Model file for the job. Use its own axes, mm. Face numbers are marked on the shaded views. A direction names the side the tool comes from. Round coordinates to 2 decimals unless told otherwise and drop trailing zeros. Write each loop counter-clockwise with the first axis right and the second up, starting at its lowest first coordinate (ties: lowest second). Pieces come first, ordered by that corner, then holes. Notation, with made-up numbers: (41.25, 45.25) - (75.25, 45.25) arc R26 cw to (75.25, 81.25) - close; hole circle Ø2 at (87, -18). An arc over 180 degrees is marked (long way). One line per item, written item: value.
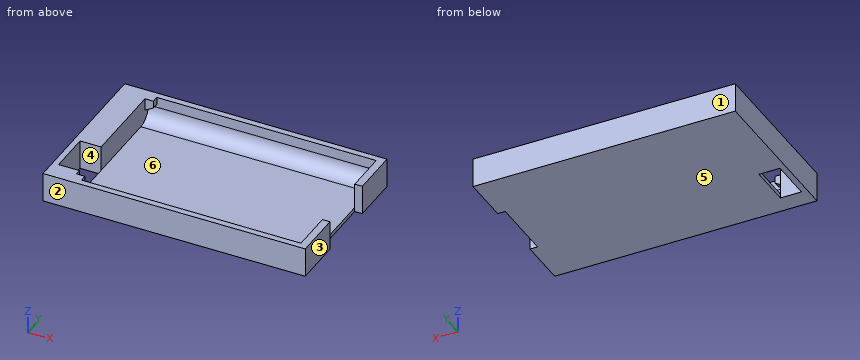
from build123d import *

# Parameters (mm, degrees)
SKETCH2_W                 = 62.4
SKETCH2_H                 = 38
BOSS_EXTRUDE1_DEPTH       = 7
CUT_EXTRUDE1_DEPTH        = 27.1
SKETCH4_W                 = 1.8
SKETCH4_H                 = 15
FORFINGER_DEPTH           = 40.143965052
SKETCH5_W                 = 2
SKETCH5_H                 = 2.9
BOSS_EXTRUDE2_DEPTH       = 1.6
CHAMFER1_SIZE2            = 1.154700538
CHAMFER1_SIZE             = 2
CHAMFER1_OF_MIRROR1_SIZE2 = 1.154700538
CHAMFER1_OF_MIRROR1_SIZE  = 2
SKETCH6_W                 = 5
SKETCH6_H                 = 10
CUT_EXTRUDE3_DEPTH        = 40.143965052


with BuildPart() as part:
    # Sketch2 → Boss-Extrude1 (new body)
    with BuildSketch(Plane.XY):
        with Locations((-2.3, 0)):
            Rectangle(SKETCH2_W, SKETCH2_H)
    extrude(amount=BOSS_EXTRUDE1_DEPTH)

    # Sketch3 → Cut-Extrude1 (cut, symmetric)
    with BuildSketch(Plane(origin=(0, 0, 0), x_dir=(0, 0, -1), z_dir=(1, 0, 0))):
        with BuildLine():
            Line((-8, 17.5), (-4.5, 17.5))
            ThreePointArc((-4.5, 17.5), (-2.025126266, 16.474873734), (-1, 14))
            Line((-1, 14), (-1, -14))
            ThreePointArc((-1, -14), (-2.025126266, -16.474873734), (-4.5, -17.5))
            Line((-4.5, -17.5), (-8, -17.5))
            Line((-8, -17.5), (-8, 17.5))
        make_face()
    extrude(amount=CUT_EXTRUDE1_DEPTH, both=True, mode=Mode.SUBTRACT)

    # Sketch4 → ForFinger (cut, through all)
    with BuildSketch(Plane.XY.offset(7)):
        with Locations((28, 0)):
            Rectangle(SKETCH4_W, SKETCH4_H)
    extrude(amount=-FORFINGER_DEPTH, mode=Mode.SUBTRACT)

    # Sketch5 → Boss-Extrude2 (add)
    with BuildSketch(Plane.XZ.offset(-17.5)):
        with Locations((-26.1, 5.55)):
            Rectangle(SKETCH5_W, SKETCH5_H)
    boss_extrude2 = extrude(amount=BOSS_EXTRUDE2_DEPTH)

    # Chamfer1
    chamfer1_edges = [part.edges().sort_by_distance(p)[0] for p in [
        (-25.1, 16.688533865, 4.1),
    ]]
    chamfer1_side = [part.faces().sort_by_distance(p)[0] for p in [
        (-25.123094011, 16.688533865, 4.1),
    ]]
    chamfer(chamfer1_edges, length=CHAMFER1_SIZE - 0.0001, length2=CHAMFER1_SIZE2 - 0.0001, reference=chamfer1_side[0])  # a hair under: the kernel refuses the full size

    # Mirror1: Boss-Extrude2 across plane
    add(boss_extrude2.mirror(Plane.ZX))

    # Chamfer1 of Mirror1
    chamfer1_of_mirror1_edges = [part.edges().sort_by_distance(p)[0] for p in [
        (-25.1, -16.688533865, 4.1),
    ]]
    chamfer1_of_mirror1_side = [part.faces().sort_by_distance(p)[0] for p in [
        (-25.123094011, -16.688533865, 4.1),
    ]]
    chamfer(chamfer1_of_mirror1_edges, length=CHAMFER1_OF_MIRROR1_SIZE - 0.0001, length2=CHAMFER1_OF_MIRROR1_SIZE2 - 0.0001, reference=chamfer1_of_mirror1_side[0])  # a hair under: the kernel refuses the full size

    # Sketch6 → Cut-Extrude3 (cut, through all)
    with BuildSketch(Plane.XY.offset(7)):
        with Locations((-29.6, -9.5)):
            Rectangle(SKETCH6_W, SKETCH6_H)
    extrude(amount=-CUT_EXTRUDE3_DEPTH, mode=Mode.SUBTRACT)


solid = part.part
1. Wall check: probe 1 along Y at (x, z) = (-6.5, 4.25); probe 2 along X at (y, z) = (15, 6); probe 3 along X at (y, z) = (-17, 5.75). Give the ranges that are in metal, low to high. Write a range as [from, to].
Report:
probe 1: [-19, -17.49], [17.49, 19]
probe 2: [-33.5, -27.1], [27.1, 28.9]
probe 3: [-33.5, -25.1], [27.1, 28.9]
2. Tool access for the marked faces 5 and 6: list every direction of +Z, -Z, +X, -X, +Y, -Y with a clear straight run to the whole face (end or side of a thin tool).
Report:
face 5: -Z, +X, -X, +Y, -Y
face 6: +Z
3. Band-saw the part on D-D on z = 3. Write the cut outline in (x, y), plus the area to 3 significant figures.
Report:
outline: (-33.5, -19) - (28.9, -19) - (28.9, -7.5) - (27.1, -7.5) - (27.1, -17.16) - (-27.1, -17.16) - (-27.1, -14.5) - (-32.1, -14.5) - (-32.1, -4.5) - (-27.1, -4.5) - (-27.1, 17.16) - (27.1, 17.16) - (27.1, 7.5) - (28.9, 7.5) - (28.9, 19) - (-33.5, 19) - close
area: 434 mm²
4. Mould opens along Y. For the marked faces 1, 2, 3 and 4 say: released by +Y, released by -Y, zero draft, split by the parting line, or undercut.
Report:
face 1: released by +Y
face 2: released by -Y
face 3: zero draft
face 4: undercut
5. Band-saw the part on A-A on x = 0.5. Write the cut outline in (y, z), plus the area to 3 significant figures.
Report:
outline: (-19, 0) - (19, 0) - (19, 7) - (17.5, 7) - (17.5, 4.5) arc R3.5 cw to (14, 1) - (-14, 1) arc R3.5 cw to (-17.5, 4.5) - (-17.5, 7) - (-19, 7) - close
area: 61.3 mm²
6. Band-saw the part on B-B on y = 11.5. Write the cut outline in (x, z).
Report:
outline: (-33.5, 0) - (28.9, 0) - (28.9, 7) - (27.1, 7) - (27.1, 1) - (-27.1, 1) - (-27.1, 7) - (-33.5, 7) - close
7. Band-saw the part on C-C on x = -28.5. Write the cut outline in (y, z), plus the area to 3 significant figures.
Report:
outline: (-19, 0) - (-14.5, 0) - (-14.5, 7) - (-19, 7) - close; (-4.5, 0) - (19, 0) - (19, 7) - (-4.5, 7) - close
area: 196 mm²
